Could you check a few things on this model? Use its own coordinates, in mm. Face numbers are marked on the shaded views. Give positions to 0.01 mm unless a question says otherwise; leave off trailing zeros. Write each loop counter-clockwise with the first axis right and the second up, starting at its lowest first coordinate (ties: lowest second). Pieces come first, ordered by that corner, then holes. Notation, with made-up numbers: M 22,37 L 35,37 A14 ccw 35,44 Z; hole C -38.5,-20.75 d7. An arc over 180 degrees is marked long. One line per item, written item: value.
```python
from build123d import *

# Parameters (mm, degrees)
SKETCH1_W              = 1397
SKETCH1_H              = 127
BOSS_EXTRUDE1_DEPTH    = 9.525
CUT_EXTRUDE1_DEPTH     = 702.445098083
F_10_CLEARANCE_HOLE1_D = 5.6134
CUT_EXTRUDE2_REACH     = 703.445
SKETCH8_R              = 7.9375


with BuildPart() as part:
    # Sketch1 → Boss-Extrude1 (new body)
    with BuildSketch(Plane.XY):
        Rectangle(SKETCH1_W, SKETCH1_H)
    extrude(amount=-BOSS_EXTRUDE1_DEPTH)

    # Sketch2 → Cut-Extrude1 (cut, through all)
    with BuildSketch(Plane.XY):
        with BuildLine():
            Line((-579.4375, -63.5), (579.4375, -63.5))
            Line((579.4375, -63.5), (579.4375, -30.1625))
            ThreePointArc((579.4375, -30.1625), (578.50756403, -27.91743597), (576.2625, -26.9875))
            Line((576.2625, -26.9875), (-576.2625, -26.9875))
            ThreePointArc((-576.2625, -26.9875), (-578.50756403, -27.91743597), (-579.4375, -30.1625))
            Line((-579.4375, -30.1625), (-579.4375, -63.5))
        make_face()
    extrude(amount=-CUT_EXTRUDE1_DEPTH, mode=Mode.SUBTRACT)

    # #10 Clearance Hole1 (through all)
    with Locations(Plane.XY):
        with Locations((-692.15, 6.35), (-692.15, -50.8), (692.15, 6.35), (692.15, -50.8), (-565.15, -14.2875), (-241.3, -14.2875), (0, -14.2875), (241.3, -14.2875), (565.15, -14.2875)):
            Hole(F_10_CLEARANCE_HOLE1_D / 2)

    # Sketch8 → Cut-Extrude2 (cut, up to next)
    with BuildSketch(Plane.XY, mode=Mode.PRIVATE) as cut_extrude2_sk1:
        with Locations((-431.8, -7.9375)):
            Circle(SKETCH8_R)
    cut_extrude2_tool1 = extrude(cut_extrude2_sk1.sketch, amount=-CUT_EXTRUDE2_REACH, mode=Mode.PRIVATE) & part.part
    # Sketch8 → Cut-Extrude2 (cut, up to next)
    with BuildSketch(Plane.XY, mode=Mode.PRIVATE) as cut_extrude2_sk2:
        with Locations((-279.4, -7.9375)):
            Circle(SKETCH8_R)
    cut_extrude2_tool2 = extrude(cut_extrude2_sk2.sketch, amount=-CUT_EXTRUDE2_REACH, mode=Mode.PRIVATE) & part.part
    # Sketch8 → Cut-Extrude2 (cut, up to next)
    with BuildSketch(Plane.XY, mode=Mode.PRIVATE) as cut_extrude2_sk3:
        with Locations((279.4, -7.9375)):
            Circle(SKETCH8_R)
    cut_extrude2_tool3 = extrude(cut_extrude2_sk3.sketch, amount=-CUT_EXTRUDE2_REACH, mode=Mode.PRIVATE) & part.part
    # Sketch8 → Cut-Extrude2 (cut, up to next)
    with BuildSketch(Plane.XY, mode=Mode.PRIVATE) as cut_extrude2_sk4:
        with Locations((431.8, -7.9375)):
            Circle(SKETCH8_R)
    cut_extrude2_tool4 = extrude(cut_extrude2_sk4.sketch, amount=-CUT_EXTRUDE2_REACH, mode=Mode.PRIVATE) & part.part
    add(cut_extrude2_tool1.solids().sort_by_distance((-431.8, -7.9375, 0))[0], mode=Mode.SUBTRACT)
    add(cut_extrude2_tool2.solids().sort_by_distance((-279.4, -7.9375, 0))[0], mode=Mode.SUBTRACT)
    add(cut_extrude2_tool3.solids().sort_by_distance((279.4, -7.9375, 0))[0], mode=Mode.SUBTRACT)
    add(cut_extrude2_tool4.solids().sort_by_distance((431.8, -7.9375, 0))[0], mode=Mode.SUBTRACT)


solid = part.part
```
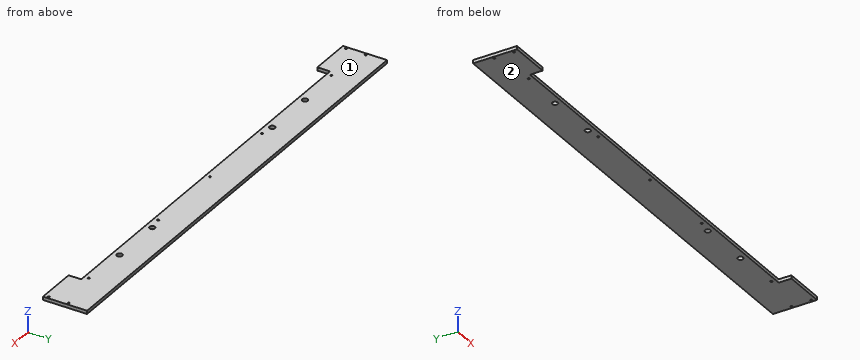
1) If we section it at A-A, the plane z = -7.5: Give the number of separate pieces and of enclosed holes in the cut face, then the cut area to 3 significant figures.
Outcome:
separate pieces: 1
enclosed holes: 13
area: 134,000 mm^2
2) If we section it at B-B, the plane x = 346.5: Write out the boundary of the cut face in (y, z) (1 decimal).
Outcome:
outline: M -27,-9.5 L 63.5,-9.5 L 63.5,0 L -27,0 Z
3) We'd pull the mould along Z, two halves only. Please class the marked faces 1 and 2: pulls with the +Z half, pulls with the -Z half, needs draft (parallel to the pull), parting line crosses it, or undercut.
Outcome:
face 1: pulls with the +Z half
face 2: pulls with the -Z half
4) Please list where these lines run through material, in increasing order: L1, parallel to Y at x = 692.15, z = -2.75; L2, parallel to X at y = -50.5, z = -0.25; L3, parallel to X at y = -44, z = -1. Write a range as from..to.
Outcome:
L1: y = -63.5..-53.61, -47.99..3.54, 9.16..63.5
L2: x = -698.5..-694.94, -689.36..-579.44, 579.44..689.36, 694.94..698.5
L3: x = -698.5..-579.44, 579.44..698.5
